from build123d import *

# Parameters (mm, degrees)
SCHIZZO1_R                   = 7
ESTRUSIONE_ESTRUSIONE1_DEPTH = 30
SMUSSO1_SIZE                 = 1
SCHIZZO6_R                   = 10.5
ESTRUSIONE_ESTRUSIONE3_DEPTH = 14
TAGLIO_ESTRUSIONE3_DEPTH     = 10
SCHIZZO8_R                   = 6.92820323
TAGLIO_ESTRUSIONE4_DEPTH     = 1
TAGLIO_ESTRUSIONE4_TAPER     = 43
RACCORDO5_R                  = 0.5
SCHIZZO9_R                   = 13.5
SCHIZZO9_R_2                 = 10.5
ESTRUSIONE_ESTRUSIONE4_DEPTH = 2
RACCORDO6_R                  = 0.2


with BuildPart() as part:
    # Schizzo1 → Estrusione-Estrusione1 (new body)
    with BuildSketch(Plane.XY):
        Circle(SCHIZZO1_R)
    extrude(amount=ESTRUSIONE_ESTRUSIONE1_DEPTH)

    # Smusso1
    smusso1_edges = [part.edges().sort_by_distance(p)[0] for p in [
        (-7, 0, 0),
    ]]
    chamfer(smusso1_edges, length=SMUSSO1_SIZE)

    # Schizzo6 → Estrusione-Estrusione3 (add)
    with BuildSketch(Plane.XY.offset(30)):
        Circle(SCHIZZO6_R)
    extrude(amount=ESTRUSIONE_ESTRUSIONE3_DEPTH)

    # Schizzo7 → Taglio-Estrusione3 (cut)
    with BuildSketch(Plane.XY.offset(44)):
        Polygon((3.464101615, 6), (-3.464101615, 6), (-6.92820323, 0), (-3.464101615, -6), (3.464101615, -6), (6.92820323, 0), align=None)
    extrude(amount=-TAGLIO_ESTRUSIONE3_DEPTH, mode=Mode.SUBTRACT)

    # Schizzo8 → Taglio-Estrusione4 (cut)
    with BuildSketch(Plane.XY.offset(44)):
        Circle(SCHIZZO8_R)
    extrude(amount=-TAGLIO_ESTRUSIONE4_DEPTH, taper=TAGLIO_ESTRUSIONE4_TAPER, mode=Mode.SUBTRACT)

    # Raccordo5
    raccordo5_edges = [part.edges().sort_by_distance(p)[0] for p in [
        (-10.5, 0, 44),
    ]]
    fillet(raccordo5_edges, radius=RACCORDO5_R)

    # Schizzo9 → Estrusione-Estrusione4 (add)
    with BuildSketch(Plane(origin=(0, 0, 30), x_dir=(-1, 0, 0), z_dir=(0, 0, -1))):
        Circle(SCHIZZO9_R)
        Circle(SCHIZZO9_R_2, mode=Mode.SUBTRACT)
    extrude(amount=-ESTRUSIONE_ESTRUSIONE4_DEPTH)

    # Raccordo6
    raccordo6_edges = [part.edges().sort_by_distance(p)[0] for p in [
        (-10.5, 0, 32),
        (13.5, 0, 32),
        (13.5, 0, 30),
    ]]
    fillet(raccordo6_edges, radius=RACCORDO6_R)


solid = part.part
Geometry check sheet. Reference: the model listing, model coordinates, mm. A direction names the side the tool comes from. Coordinates: 2 decimals unless noted, no trailing zeros. Order: outer loops, then holes, each group sorted by start corner. A loop starts at its lowest first (then second) coordinate and runs counter-clockwise, first axis right, second up. Notation, with made-up numbers: (52.25, -27) - (78.25, -27) arc R17 cw to (78.25, -4) - close; hole circle Ø2 at (33, 38). An arc over 180 degrees is marked (long way). Answer in a Markdown table with one row per item. Add a question column.
1) Release check for a two-part mould opening along X. For faces 1 (the cylindrical face through (6.466, -2.681, 15.297)), 2 (the flat face through (-2, -7, 44)), 3 (the flat face through (5.22, 2.96, 39.07)) record: +X half, -X half, draft (parallel to the pull), parting line (faces both ways), or undercut.
2) Gauge pin test, flat ends, axial feed: P1, Ø8, axis at x = 10.5, z = 34, coming from the -Y side; P2, Ø8, axis at y = 9, z = 24, coming from the +X side; P3, Ø3, axis at x = -5, z = 23.5, coming from the +Y side. Record the tip position at first contact, or that the pin passes through.
3) Cross-section at A-A, the plane x = 0. Record the cut outline in (y, z).
4) Set-up check for faces 4 (the flat face through (-6, -6, 30)), 5 (the flat face through (0, 0, 0)), 6 (the conical face through (-0.05, -6.46, 43.5)): record each of +Z, -Z, +X, -X, +Y, -Y from which the full face is reachable in a straight line by a thin tool's end or side.
5) Material ranges on line 1 along X through (y, z) = (-1, 12); line 2 along Z through (x, y) = (2, -1.25); line 3 along Z through (x, y) = (-4.5, -5.5), recorded low to high. Write a range as [from, to].
6) Cross-section at B-B, the plane z = 14. Record the cut outline in (x, y), then the cut area to 3 significant figures.
Check result:
| question | item | result |
|---|---|---|
| 1 | face 1 | parting line |
| 1 | face 2 | draft |
| 1 | face 3 | undercut |
| 2 | P1 | stops at y = -11.46 |
| 2 | P2 | stops at x = 4.9 |
| 2 | P3 | stops at y = 6.06 |
| 3 | outline | (-13.5, 30.2) arc R0.2 ccw to (-13.3, 30) - (-7, 30) - (-7, 1) - (-6, 0) - (6, 0) - (7, 1) - (7, 30) - (13.3, 30) arc R0.2 ccw to (13.5, 30.2) - (13.5, 31.8) arc R0.2 ccw to (13.3, 32) - (10.7, 32) arc R0.2 cw to (10.5, 32.2) - (10.5, 43.5) arc R0.5 ccw to (10, 44) - (6.93, 44) - (6, 43) - (6, 34) - (-6, 34) - (-6, 43) - (-6.93, 44) - (-10, 44) arc R0.5 ccw to (-10.5, 43.5) - (-10.5, 32.2) arc R0.2 cw to (-10.7, 32) - (-13.3, 32) arc R0.2 ccw to (-13.5, 31.8) - close |
| 4 | face 4 | -Z |
| 4 | face 5 | -Z, +X, -X, +Y, -Y |
| 4 | face 6 | +Z |
| 5 | line 1 | x = [-6.93, 6.93] |
| 5 | line 2 | z = [0, 34] |
| 5 | line 3 | z = [30, 44] |
| 6 | outline | circle Ø14 at (0, 0) |
| 6 | area | 154 mm² |
